Part model, mm, in its own coordinate system. Face numbers are marked on the shaded views. A direction names the side the tool comes from. Round coordinates to 2 decimals unless told otherwise and drop trailing zeros. Loops run counter-clockwise (first coordinate to the right, second up) from the corner with the lowest first, then second, coordinate; pieces in that order, holes last.
(1) Mould opens along Y. For the marked faces 1, 2, 3 and 4 say: +Y half, -Y half, draft (parallel to the pull), parting line (faces both ways), or undercut.
(2) Cut at A-A on z = 16. List the corners of the cut face in (x, y).
(3) Tool access for the marked faces 5 and 6: list every direction of +Z, -Z, +X, -X, +Y, -Y with a clear straight run to the whole face (end or side of a thin tool).
(4) Cut at D-D on z = 9.5. List the corners of the cut face in (x, y), then the cut area to 3 significant figures.
(5) Cut at C-C on x = 15. List the corners of the cut face in (y, z).
(6) Probe probe 1 along Y at (x, z) = (31.5, 20); probe 2 along Z at (x, y) = (26, -33); probe 3 along X at (y, z) = (-16, 24.5). List the from-to ranges inside material, lowest first.
(7) Cut at B-B on y = -11. List the corners of the cut face in (x, z), then the cut area to 3 significant figures.
(8) Flat gauge pin, fed straight in: pin 1 (1.5 mm diameter, centred on y = -32, z = 28.5, fed in from +X). Where does the tip first touch, or does it go through?
from build123d import *

# Parameters (mm, degrees)
F0_W     = 28.295456
F0_H     = 30
F1_DEPTH = 50
F2_R     = 5.08
F3_T     = -2.54
F4_R     = 8
F5_DEPTH = 9.1


with BuildPart() as f1:
    # F0 (on Front) → F1 (new body)
    with BuildSketch(Plane.XZ):
        with Locations((20.883416, 19.067463)):
            Rectangle(F0_W, F0_H)
    extrude(amount=F1_DEPTH)

    # F2
    f2_edges = [f1.edges().sort_by_distance(p)[0] for p in [
        (20.883416, -50, 34.067463),
    ]]
    fillet(f2_edges, radius=F2_R)

    # F3
    f3_openings = [f1.faces().sort_by_distance(p)[0] for p in [
        (35.031144, -24.911561, 19.016082),
    ]]
    offset(amount=F3_T, openings=f3_openings)

    # F4 (on face) → F5 (cut)
    with BuildSketch(Plane.YZ.offset(9.275688)):
        with Locations((-33.887234, 21.420674)):
            Circle(F4_R)
    extrude(amount=-F5_DEPTH, mode=Mode.SUBTRACT)


solid = f1.part
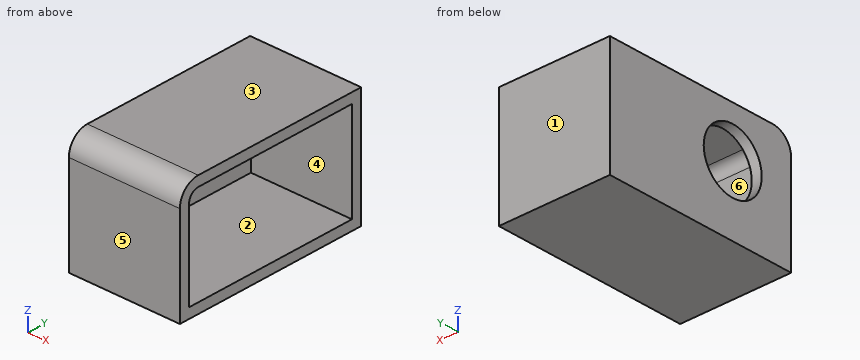
Final values:
1. face 1: +Y half
1. face 2: undercut
1. face 3: draft
1. face 4: undercut
2. outline: (6.74, -50) - (35.03, -50) - (35.03, -47.46) - (9.28, -47.46) - (9.28, -39.77) - (6.74, -39.77) - close; (6.74, -28) - (9.28, -28) - (9.28, -2.54) - (35.03, -2.54) - (35.03, 0) - (6.74, 0) - close
3. face 5: +Z, -Z, +X, -X, -Y
3. face 6: +X
4. outline: (6.74, -50) - (35.03, -50) - (35.03, -47.46) - (9.28, -47.46) - (9.28, -2.54) - (35.03, -2.54) - (35.03, 0) - (6.74, 0) - close
4. area: 258 mm2
5. outline: (-50, 4.07) - (0, 4.07) - (0, 34.07) - (-44.92, 34.07) arc R5.08 ccw to (-50, 28.99) - close; hole (-47.46, 6.61) - (-2.54, 6.61) - (-2.54, 31.53) - (-44.92, 31.53) arc R2.54 ccw to (-47.46, 28.99) - close
6. probe 1: y = -50 to -47.46, -2.54 to 0
6. probe 2: z = 4.07 to 6.61, 31.53 to 34.07
6. probe 3: x = 6.74 to 9.28
7. outline: (6.74, 4.07) - (35.03, 4.07) - (35.03, 6.61) - (9.28, 6.61) - (9.28, 31.53) - (35.03, 31.53) - (35.03, 34.07) - (6.74, 34.07) - close
7. area: 207 mm2
8. pin 1: stops at x = 9.28
